Verification items for this drawing (mm, ordinates from the low corner). A direction names the side the tool comes from. Round coordinates to 2 decimals unless told otherwise and drop trailing zeros. Loops run counter-clockwise (first coordinate to the right, second up) from the corner with the lowest first, then second, coordinate; pieces in that order, holes last. Notation, with made-up numbers: M -17.75,34.5 L 36.25,34.5 A21 cw 36.25,41.5 Z; hole C 22,49 d9. An arc over 180 degrees is marked long. Write item = value, one per line.
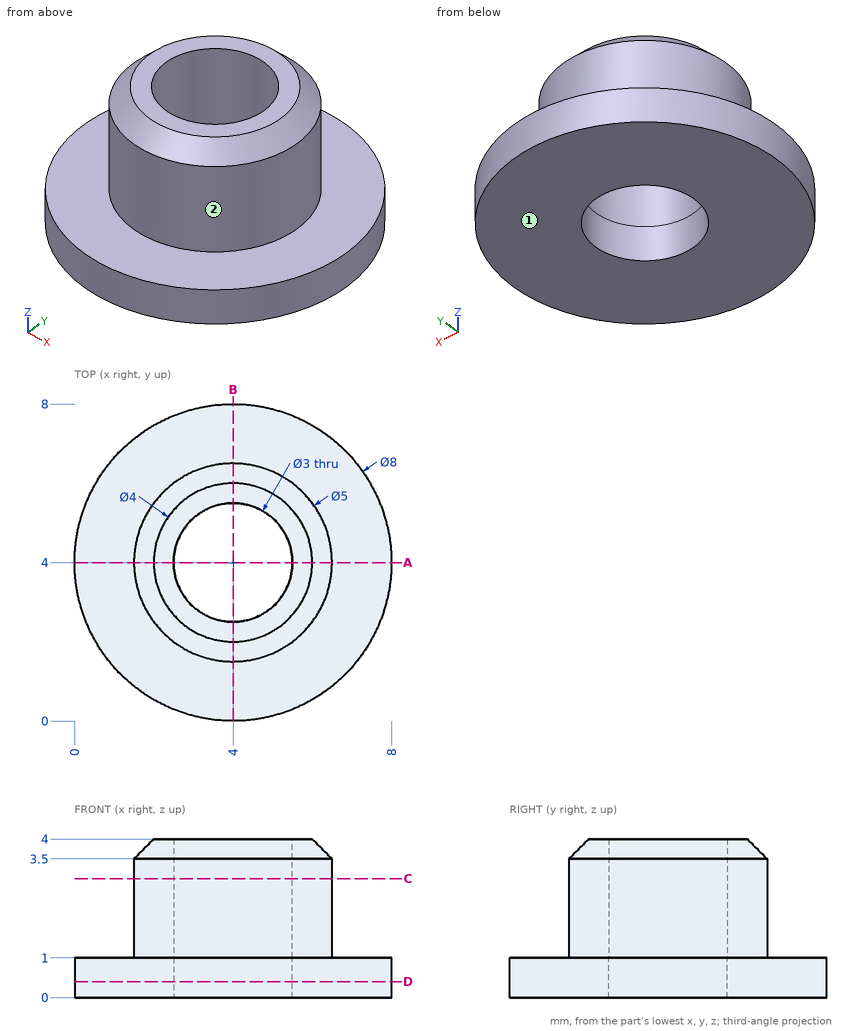
(1) Depth check by flat-ended pin: pin 1 Ø1 at (y, z) = (4, 2.5) entering from -X; pin 2 Ø1.5 at (y, z) = (2.5, 2) entering from +X. Enter the tip coordinate at first touch or a pass-through.
Result set:
pin_1 = 1.5
pin_2 = 6.38
(2) Tool access check on the marked faces 1 and 2. Record the directions out of +Z, -Z, +X, -X, +Y, -Y that give a thin tool (end or side, any length) a straight path to the whole face; none if there is none.
Result set:
face_1 = -Z, +X, -X, +Y, -Y
face_2 = +Z
(3) Sectioned sample at A-A on y = 4. Record the cut outline in (x, z).
Result set:
outline = M 0,0 L 2.5,0 L 2.5,4 L 2,4 L 1.5,3.5 L 1.5,1 L 0,1 Z; M 5.5,0 L 8,0 L 8,1 L 6.5,1 L 6.5,3.5 L 6,4 L 5.5,4 Z
(4) Sectioned sample at C-C on z = 3. Record the cut outline in (x, y), then the cut area to 3 significant figures.
Result set:
outline = C 4,4 d5; hole C 4,4 d3
area = 12.6 mm2
(5) Sectioned sample at D-D on z = 0.4. Record the cut outline in (x, y).
Result set:
outline = C 4,4 d8; hole C 4,4 d3
(6) Material ranges on line 1 along Y through (x, z) = (4, 0.3); line 2 along Y through (x, z) = (4, 2.9); line 3 along X through (y, z) = (6, 2.7), recorded low to high. Write a range as from..to.
Result set:
line_1 = 0..2.5, 5.5..8
line_2 = 1.5..2.5, 5.5..6.5
line_3 = 2.5..5.5
